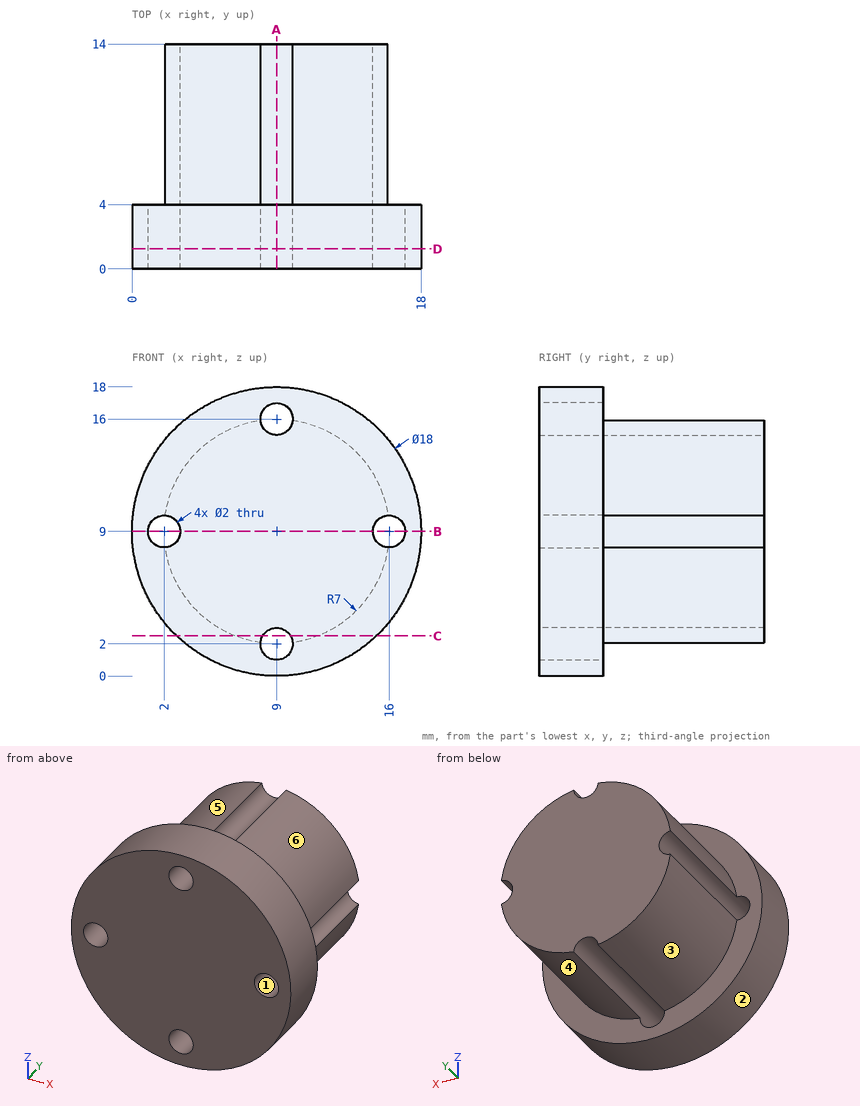
Source: three-view drawing plus pictorial views. Frame: mm from the lowest corner of the part. A direction names the side the tool comes from. Give positions to 0.01 mm unless a question says otherwise; leave off trailing zeros. Order: outer loops, then holes, each group sorted by start corner. A loop starts at its lowest first (then second) coordinate and runs counter-clockwise, first axis right, second up. Notation, with made-up numbers: M 32,-20 L 76,-20 A14 cw 76,-10 Z; hole C 34.25,88.25 d8. An arc over 180 degrees is marked long. Return JSON: item names as keys, results as strings.
Item 1: Access query for the marked faces 4, 5 and 6. Directions: +Z, -Z, +X, -X, +Y, -Y. A direction counts if a zero-diameter tool reaches every point of the face in a straight line with its end or side. Return the directions, or none.
Solutions:
{"face 4": "-Z, +X, +Y", "face 5": "+Z, -X, +Y", "face 6": "+Z, +X, +Y"}
Item 2: Ray query, probe 1 along X at (y, z) = (3.5, 9.75); probe 2 along Z at (x, y) = (9, 9). Return the intervals inside material, ascending.
Solutions:
{"probe 1": "0.03 to 1.34, 2.66 to 15.34, 16.66 to 17.97", "probe 2": "3 to 15"}
Item 3: Cut plane C-C (z = 2.5). Return loops of the section in (x, y).
Solutions:
{"outline": "M 2.78,0 L 8.13,0 L 8.13,14 L 6.4,14 L 6.4,4 L 2.78,4 Z; M 9.87,0 L 15.22,0 L 15.22,4 L 11.6,4 L 11.6,14 L 9.87,14 Z"}
Item 4: Cut plane A-A (x = 9). Return loops of the section in (y, z), then the cut area to 3 significant figures.
Solutions:
{"outline": "M 0,0 L 4,0 L 4,1 L 0,1 Z; M 0,3 L 14,3 L 14,15 L 0,15 Z; M 0,17 L 4,17 L 4,18 L 0,18 Z", "area": "176 mm^2"}
Item 5: Cut plane D-D (y = 1.25). Return loops of the section in (x, z), then the cut area to 3 significant figures.
Solutions:
{"outline": "C 9,9 d18; hole C 2,9 d2; hole C 9,2 d2; hole C 9,16 d2; hole C 16,9 d2", "area": "242 mm^2"}
Item 6: Pull-direction query (Z, two-part tool) for the marked faces 1, 2 and 3; classes: +Z half, -Z half, draft (parallel to the pull), parting line (faces both ways), or undercut.
Solutions:
{"face 1": "undercut", "face 2": "parting line", "face 3": "-Z half"}
Item 7: First-contact query: P1, Ø2, axis at y = 8.5, z = 10, coming from the -X side; P2, Ø1.5, axis at x = 5.5, y = 5.5, coming from the -Z side; P3, Ø1, axis at x = 8, y = 11, coming from the +Z side. Flat tips, straight axial feed; report the tip coordinate or a pass-through.
Solutions:
{"P1": "x = 2.07", "P2": "z = 2.56", "P3": "z = 15.93"}
Item 8: Cut plane B-B (z = 9). Return loops of the section in (x, y), then the cut area to 3 significant figures.
Solutions:
{"outline": "M 0,0 L 1,0 L 1,4 L 0,4 Z; M 3,0 L 15,0 L 15,14 L 3,14 Z; M 17,0 L 18,0 L 18,4 L 17,4 Z", "area": "176 mm^2"}
